Could you check a few things on this model? Use its own coordinates, in mm. A direction names the side the tool comes from. Round coordinates to 2 decimals unless told otherwise and drop trailing zeros. Loops run counter-clockwise (first coordinate to the right, second up) from the corner with the lowest first, then second, coordinate; pieces in that order, holes last. Notation, with made-up numbers: (-33.5, -23) -> (19.5, -23) arc R10 ccw to (19.5, -11) -> close; hole circle Ø1 at (66, 22.5). An arc over 180 degrees is marked (long way). One line per item, written item: value.
```python
from build123d import *

# Parameters (mm, degrees)
SKETCH_R           = 10
PAD_DEPTH          = 15
POCKET_DEPTH       = 15.001
POCKET001_DEPTH    = 79.032242
POLARPATTERN_COUNT = 12


with BuildPart() as part:
    # Sketch → Pad (new body)
    with BuildSketch(Plane.XY):
        Circle(SKETCH_R)
    extrude(amount=PAD_DEPTH)

    # Sketch001 (on Face3 of Pad) → Pocket (cut, through all)
    with BuildSketch(Plane.XY.offset(15)):
        with BuildLine():
            ThreePointArc((2.575, 1.857418), (-3.175, 0), (2.575, -1.857418))
            Line((2.575, 1.857418), (2.575, -1.857418))
        make_face()
    extrude(amount=-POCKET_DEPTH, mode=Mode.SUBTRACT)

    # Sketch002 (on Face3 of Pocket) → Pocket001 (cut, through all)
    with BuildSketch(Plane.XY.offset(15)):
        Polygon((-1, 5), (1, 5), (2.041891, 10.908846), (-2.041888, 10.908847), align=None)
    pocket001 = extrude(amount=-POCKET001_DEPTH, mode=Mode.SUBTRACT)

    # PolarPattern: Pocket001 ×12 about axis
    polarpattern_axis = Axis((0, 0, 15), (0, 0, 1))
    for i in range(1, POLARPATTERN_COUNT):
        add(pocket001.rotate(polarpattern_axis, i * 360 / POLARPATTERN_COUNT), mode=Mode.SUBTRACT)


solid = part.part
```
Item 1: For faces 1 (the face through (-2.484, -7.165, 7.605)), 2 (the face through (-5.73, -4.96, 7.6)), 3 (the face through (-1.43, 7.45, 7.6)), which set-ups out of +Z, -Z, +X, -X, +Y, -Y let a thin tool reach every point of the face, with its end or its side?
Output:
face 1: +Z, -Z
face 2: +Z, -Z, -X
face 3: +Z, -Z, +Y
Item 2: Will these pins go through, and if not, where does the flat tip stop? pin 1 Ø2 at (y, z) = (3, 5.5) entering from -X; pin 2 Ø4 at (x, z) = (-6.5, 10) entering from +Y (3 decimals); pin 3 Ø3 at (x, z) = (-6.5, 12) entering from -Y (3 decimals).
Output:
pin 1: stops at x = -9.8
pin 2: stops at y = 7.585
pin 3: stops at y = -7.585
Item 3: If we section it at D-D on y = -2.25: List the corners of the cut face in (x, z) for me, plus the area to 3 significant figures.
Output:
outline: (-9.74, 0) -> (-6.52, 0) -> (-6.52, 15) -> (-9.74, 15) -> close; (-4.47, 0) -> (-2.24, 0) -> (-2.24, 15) -> (-4.47, 15) -> close; (2.24, 0) -> (4.47, 0) -> (4.47, 15) -> (2.24, 15) -> close; (6.52, 0) -> (9.74, 0) -> (9.74, 15) -> (6.52, 15) -> close
area: 164 mm²
Item 4: If we section it at C-C on x = 4.5: List the corners of the cut face in (y, z) for me.
Output:
outline: (-5.18, 0) -> (-3.93, 0) -> (-3.93, 15) -> (-5.18, 15) -> close; (-2.21, 0) -> (2.21, 0) -> (2.21, 15) -> (-2.21, 15) -> close; (3.93, 0) -> (5.18, 0) -> (5.18, 15) -> (3.93, 15) -> close
Item 5: I need wall thicknesses on line 1 (X direction, y = -6, z = 11.75); line 2 (Y direction, x = 0, z = 11.5) (3 decimals); line 3 (X direction, y = 0, z = 6.5) (3 decimals). Which ranges of each line are inside material? Lowest first, please. Write a range as from..to.
Output:
line 1: x = -6.97..-5.19, -2.06..-1.18, 1.18..2.06, 5.19..6.97
line 2: y = -5..-3.175, 3.175..5
line 3: x = -5..-3.175, 2.575..5
Item 6: If we section it at B-B on y = 0: List the corners of the cut face in (x, z) for me (3 decimals), plus the area to 4 significant figures.
Output:
outline: (-5, 0) -> (-3.175, 0) -> (-3.175, 15) -> (-5, 15) -> close; (2.575, 0) -> (5, 0) -> (5, 15) -> (2.575, 15) -> close
area: 63.75 mm²
Item 7: If we section it at A-A on x = 0: List the corners of the cut face in (y, z) for me (3 decimals).
Output:
outline: (-5, 0) -> (-3.175, 0) -> (-3.175, 15) -> (-5, 15) -> close; (3.175, 0) -> (5, 0) -> (5, 15) -> (3.175, 15) -> close
Item 8: If we mould it in two halves opening along Y, with no side actions, what happens to faces 4 (the face through (-9.66, -2.58, 7.4)), 5 (the face through (-7.06, 7.08, 7.4)), 6 (the face through (-7.1, -2.46, 7.6))? For each: released by +Y, released by -Y, zero draft, split by the parting line, or undercut.
Output:
face 4: released by -Y
face 5: released by +Y
face 6: undercut
